Check sheet for the modelled part. Datum: model origin and axes. Units: mm. A direction names the side the tool comes from. Give positions to 0.01 mm unless a question says otherwise; leave off trailing zeros. Order: outer loops, then holes, each group sorted by start corner. A loop starts at its lowest first (then second) coordinate and runs counter-clockwise, first axis right, second up.
from build123d import *

# Parameters (mm, degrees)
SKETCH2_W           = 51
SKETCH2_H           = 101
SKETCH2_W_2         = 49
SKETCH2_H_2         = 99
BOSS_EXTRUDE2_DEPTH = 1600
SKETCH3_R           = 40.5
CUT_EXTRUDE2_DEPTH  = 52


with BuildPart() as part:
    # Sketch2 → Boss-Extrude2 (new body)
    with BuildSketch(Plane(origin=(0, 0, 0), x_dir=(1, 0, 0), z_dir=(0, 1, 0))):
        Rectangle(SKETCH2_W, SKETCH2_H)
        Rectangle(SKETCH2_W_2, SKETCH2_H_2, mode=Mode.SUBTRACT)
    extrude(amount=BOSS_EXTRUDE2_DEPTH)

    # Sketch3 → Cut-Extrude2 (cut, through all)
    with BuildSketch(Plane.ZY.offset(25.5)):
        with Locations((0, 50)):
            Circle(SKETCH3_R)
        with Locations((0, 1550)):
            Circle(SKETCH3_R)
    extrude(amount=-CUT_EXTRUDE2_DEPTH, mode=Mode.SUBTRACT)


solid = part.part
1) Section check C-C, the plane z = 26. Record the cut outline in (x, y), then the cut area to 3 significant figures.
Recorded:
outline: (-25.5, 0) - (-24.5, 0) - (-24.5, 18.95) - (-25.5, 18.95) - close; (-25.5, 81.05) - (-24.5, 81.05) - (-24.5, 1518.95) - (-25.5, 1518.95) - close; (-25.5, 1581.05) - (-24.5, 1581.05) - (-24.5, 1600) - (-25.5, 1600) - close; (24.5, 0) - (25.5, 0) - (25.5, 18.95) - (24.5, 18.95) - close; (24.5, 81.05) - (25.5, 81.05) - (25.5, 1518.95) - (24.5, 1518.95) - close; (24.5, 1581.05) - (25.5, 1581.05) - (25.5, 1600) - (24.5, 1600) - close
area: 2,950 mm2
2) Set-up check for faces 1 (the face through (-25, 1600, 0)), 2 (the face through (24.5, 789, 1)): record each of +Z, -Z, +X, -X, +Y, -Y from which the full face is reachable in a straight line by a thin tool's end or side.
Recorded:
face 1: +Z, -Z, +X, -X, +Y
face 2: +Y, -Y
3) Section check D-D, the plane y = 178.5. Record the cut outline in (x, z).
Recorded:
outline: (-25.5, -50.5) - (25.5, -50.5) - (25.5, 50.5) - (-25.5, 50.5) - close; hole (-24.5, -49.5) - (24.5, -49.5) - (24.5, 49.5) - (-24.5, 49.5) - close
4) Section check A-A, the plane y = 1550. Record the cut outline in (x, z), then the cut area to 3 significant figures.
Recorded:
outline: (-25.5, -50.5) - (25.5, -50.5) - (25.5, -40.5) - (24.5, -40.5) - (24.5, -49.5) - (-24.5, -49.5) - (-24.5, -40.5) - (-25.5, -40.5) - close; (-25.5, 40.5) - (-24.5, 40.5) - (-24.5, 49.5) - (24.5, 49.5) - (24.5, 40.5) - (25.5, 40.5) - (25.5, 50.5) - (-25.5, 50.5) - close
area: 138 mm2
5) Section check B-B, the plane x = -7. Record the cut outline in (y, z), then the cut area to 3 significant figures.
Recorded:
outline: (0, -50.5) - (1600, -50.5) - (1600, -49.5) - (0, -49.5) - close; (0, 49.5) - (1600, 49.5) - (1600, 50.5) - (0, 50.5) - close
area: 3,200 mm2
6) Material ranges on L1, parallel to Y at x = -25.05, z = 0; L2, parallel to X at y = 1077.5, z = -41.5; L3, parallel to Z at x = 24, y = 50, recorded low to high.
Recorded:
L1: y = 0 to 9.5, 90.5 to 1509.5, 1590.5 to 1600
L2: x = -25.5 to -24.5, 24.5 to 25.5
L3: z = -50.5 to -49.5, 49.5 to 50.5
7) Draft check along Y on faces 3 (the face through (-25, 0, 0)), 4 (the face through (24.993, 90.155, -5.272)), 5 (the face through (-24.5, 789, 1)). Enter one of: +Y half, -Y half, draft (parallel to the pull), parting line (faces both ways), or undercut.
Recorded:
face 3: -Y half
face 4: undercut
face 5: draft
